Read the model definition and answer for the solid it produces. Units are mm, in the model's axes. Face numbers are marked on the shaded views. A direction names the side the tool comes from. Coordinates: 2 decimals unless noted, no trailing zeros. Loops run counter-clockwise (first coordinate to the right, second up) from the corner with the lowest first, then second, coordinate; pieces in that order, holes last. Notation, with made-up numbers: M 66,-13 L 103,-13 A18 cw 103,21 Z; hole C 47,-20 d6. An arc over 180 degrees is marked long. One line per item, written item: value. Start each with the question number.
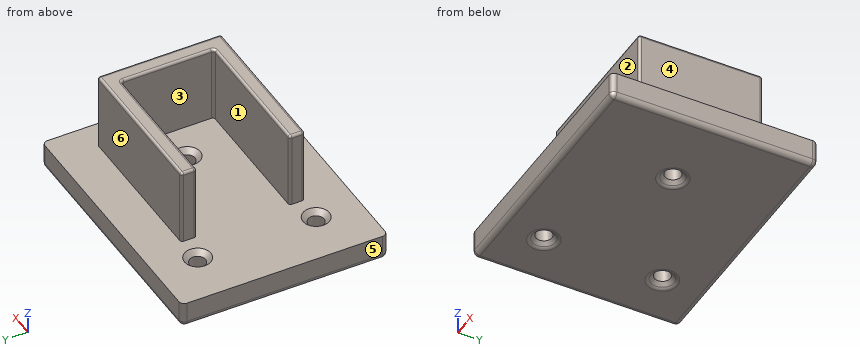
```python
from build123d import *

# Parameters (mm, degrees)
SKETCH_2_W          = 50
SKETCH_2_H          = 40
EXTRUDE_1_DEPTH     = 5
EXTRUDE_START       = -8
SKETCH_5_W          = 30
SKETCH_5_H          = 15
EXTRUDE_2_DEPTH     = 3
SKETCH_6_W          = 30
SKETCH_6_H          = 15
EXTRUDE_3_DEPTH     = 3
CUT_EXTRUDE_1_REACH = 39.749
SKETCH_7_R          = 1.55
SKETCH_8_W          = 15
SKETCH_8_H          = 21
EXTRUDE_4_DEPTH     = 3
FILLET_4_R          = 0.5
CHAMFER_1_SIZE      = 1
FILLET_3_R          = 1


with BuildPart() as part:
    # 草图2 → 凸台-拉伸1 (new body)
    with BuildSketch(Plane.XY):
        Rectangle(SKETCH_2_W, SKETCH_2_H)
    extrude(amount=EXTRUDE_1_DEPTH)

    # 草图5 → 凸台-拉伸2 (add)
    with BuildSketch(Plane.XZ.offset(20).offset(EXTRUDE_START)):
        with Locations((5, 12.5)):
            Rectangle(SKETCH_5_W, SKETCH_5_H)
    extrude(amount=-EXTRUDE_2_DEPTH)

    # 草图6 → 凸台-拉伸3 (add)
    with BuildSketch(Plane(origin=(0, 20, 0), x_dir=(1, 0, 0), z_dir=(0, 1, 0)).offset(EXTRUDE_START)):
        with Locations((5, -12.5)):
            Rectangle(SKETCH_6_W, SKETCH_6_H)
    extrude(amount=-EXTRUDE_3_DEPTH)

    # 草图7 → 切除-拉伸1 (cut, up to next)
    with BuildSketch(Plane(origin=(0, 0, 0), x_dir=(-1, 0, 0), z_dir=(0, 0, -1)), mode=Mode.PRIVATE) as cut_extrude_1_sk1:
        with Locations((-10, 0)):
            Circle(SKETCH_7_R)
    cut_extrude_1_tool1 = extrude(cut_extrude_1_sk1.sketch, amount=-CUT_EXTRUDE_1_REACH, mode=Mode.PRIVATE) & part.part
    # 草图7 → 切除-拉伸1 (cut, up to next)
    with BuildSketch(Plane(origin=(0, 0, 0), x_dir=(-1, 0, 0), z_dir=(0, 0, -1)), mode=Mode.PRIVATE) as cut_extrude_1_sk2:
        with Locations((15, -11.5)):
            Circle(SKETCH_7_R)
    cut_extrude_1_tool2 = extrude(cut_extrude_1_sk2.sketch, amount=-CUT_EXTRUDE_1_REACH, mode=Mode.PRIVATE) & part.part
    # 草图7 → 切除-拉伸1 (cut, up to next)
    with BuildSketch(Plane(origin=(0, 0, 0), x_dir=(-1, 0, 0), z_dir=(0, 0, -1)), mode=Mode.PRIVATE) as cut_extrude_1_sk3:
        with Locations((15, 11.5)):
            Circle(SKETCH_7_R)
    cut_extrude_1_tool3 = extrude(cut_extrude_1_sk3.sketch, amount=-CUT_EXTRUDE_1_REACH, mode=Mode.PRIVATE) & part.part
    add(cut_extrude_1_tool1.solids().sort_by_distance((10, 0, 0))[0], mode=Mode.SUBTRACT)
    add(cut_extrude_1_tool2.solids().sort_by_distance((-15, -11.5, 0))[0], mode=Mode.SUBTRACT)
    add(cut_extrude_1_tool3.solids().sort_by_distance((-15, 11.5, 0))[0], mode=Mode.SUBTRACT)

    # 草图8 → 凸台-拉伸4 (add)
    with BuildSketch(Plane(origin=(20, 0, 0), x_dir=(0, 0, -1), z_dir=(1, 0, 0))):
        with Locations((-12.5, -1.5)):
            Rectangle(SKETCH_8_W, SKETCH_8_H)
    extrude(amount=-EXTRUDE_4_DEPTH)

    # 圆角4
    fillet_4_edges = [part.edges().sort_by_distance(p)[0] for p in [
        (-10, -9, 12.5),
        (-10, -10.5, 20),
        (20, 0, 20),
        (20, -12, 12.5),
        (5, -12, 20),
        (-10, -12, 12.5),
        (3.5, 9, 20),
        (-10, 9, 12.5),
        (-10, 10.5, 20),
        (-10, 12, 12.5),
        (5, 12, 20),
        (20, 12, 12.5),
        (3.5, -9, 20),
        (17, 0, 20),
        (17, -9, 12.5),
        (17, 9, 12.5),
    ]]
    fillet(fillet_4_edges, radius=FILLET_4_R)

    # 倒角1
    chamfer_1_edges = [part.edges().sort_by_distance(p)[0] for p in [
        (11.55, 0, 0),
        (11.55, 0, 5),
        (-13.45, -11.5, 0),
        (-13.45, -11.5, 5),
        (-13.45, 11.5, 0),
        (-13.45, 11.5, 5),
    ]]
    chamfer(chamfer_1_edges, length=CHAMFER_1_SIZE)

    # 圆角3
    fillet_3_edges = [part.edges().sort_by_distance(p)[0] for p in [
        (12.55, 0, 0),
        (-12.45, -11.5, 0),
        (-12.45, 11.5, 0),
        (0, -20, 0),
        (-25, 0, 0),
        (0, 20, 0),
        (25, 0, 0),
        (25, -20, 2.5),
        (-25, -20, 2.5),
        (-25, 20, 2.5),
        (25, 20, 2.5),
    ]]
    fillet(fillet_3_edges, radius=FILLET_3_R)


solid = part.part
```
1) Section D-D (z = 15.75) is taken. Determine the outline of the cut face in (x, y).
2) Section A-A (x = 10) is taken. Determine the outline of the cut face in (y, z).
3) For a pull along Y with two mould halves and no side action, classify the marked faces 1, 2, 3 and 4 as released by +Y, released by -Y, zero draft, split by the parting line, or undercut.
4) Section B-B (y = 0) is taken. Determine the outline of the cut face in (x, z), then the cut area to 3 significant figures.
5) Flat-ended cylindrical pins translate along their axes: pin 1 (4.5 mm diameter, centred on y = -4.5, z = 16, fed in from +X); pin 2 (5 mm diameter, centred on x = -15, y = -11.5, fed in from -Z); pin 3 (4.5 mm diameter, centred on y = -3, z = 10, fed in from -X). Find the tip coordinate at first contact, or state that the pin passes through.
6) Section C-C (x = -15) is taken. Determine the outline of the cut face in (y, z), then the cut area to 3 significant figures.
7) A tool of negligible diameter and unlimited length cuts with its end or side. For the marked faces 5 and 6, from which of +Z, -Z, +X, -X, +Y, -Y can it reach the whole face along a straight path? Write none if from no direction.
8) Consider line 1 along Y through (x, z) = (6, 5.75); line 2 along Y through (x, z) = (-15, 2.95); line 3 along Y through (x, z) = (10, 1.95). Determine where each line is inside the solid, lowest interval first.
Results found:
1. outline: M -10,-11.5 A0.5 ccw -9.5,-12 L 19.5,-12 A0.5 ccw 20,-11.5 L 20,11.5 A0.5 ccw 19.5,12 L -9.5,12 A0.5 ccw -10,11.5 L -10,9.5 A0.5 ccw -9.5,9 L 16.5,9 A0.5 cw 17,8.5 L 17,-8.5 A0.5 cw 16.5,-9 L -9.5,-9 A0.5 ccw -10,-9.5 Z
2. outline: M -20,1 A1 ccw -19,0 L -2.96,0 A1 ccw -2.26,0.29 L -1.55,1 L -1.55,4 L -2.55,5 L -9,5 L -9,19.5 A0.5 ccw -9.5,20 L -11.5,20 A0.5 ccw -12,19.5 L -12,5 L -20,5 Z; M 1.55,1 L 2.26,0.29 A1 ccw 2.96,0 L 19,0 A1 ccw 20,1 L 20,5 L 12,5 L 12,19.5 A0.5 ccw 11.5,20 L 9.5,20 A0.5 ccw 9,19.5 L 9,5 L 2.55,5 L 1.55,4 Z
3. face 1: undercut
3. face 2: released by -Y
3. face 3: undercut
3. face 4: zero draft
4. outline: M -25,1 A1 ccw -24,0 L 7.04,0 A1 ccw 7.74,0.29 L 8.45,1 L 8.45,4 L 7.45,5 L -25,5 Z; M 11.55,1 L 12.26,0.29 A1 ccw 12.96,0 L 24,0 A1 ccw 25,1 L 25,5 L 20,5 L 20,19.5 A0.5 ccw 19.5,20 L 17.5,20 A0.5 ccw 17,19.5 L 17,5 L 12.55,5 L 11.55,4 Z
4. area: 277 mm²
5. pin 1: stops at x = 20
5. pin 2: stops at z = 0.11
5. pin 3: stops at x = 17
6. outline: M -20,1 A1 ccw -19,0 L -14.46,0 A1 ccw -13.76,0.29 L -13.05,1 L -13.05,4 L -14.05,5 L -20,5 Z; M -9.95,1 L -9.24,0.29 A1 ccw -8.54,0 L 8.54,0 A1 ccw 9.24,0.29 L 9.95,1 L 9.95,4 L 8.95,5 L -8.95,5 L -9.95,4 Z; M 13.05,1 L 13.76,0.29 A1 ccw 14.46,0 L 19,0 A1 ccw 20,1 L 20,5 L 14.05,5 L 13.05,4 Z
6. area: 164 mm²
7. face 5: +Z, -Z, -X, +Y, -Y
7. face 6: +Z, +X, -X, +Y
8. line 1: y = -12 to -9, 9 to 12
8. line 2: y = -20 to -13.05, -9.95 to 9.95, 13.05 to 20
8. line 3: y = -20 to -1.55, 1.55 to 20
